Verification items for the finished model (mm, model axes). Face numbers are marked on the shaded views. A direction names the side the tool comes from. Round coordinates to 2 decimals unless told otherwise and drop trailing zeros. Loops run counter-clockwise (first coordinate to the right, second up) from the corner with the lowest first, then second, coordinate; pieces in that order, holes last. Notation, with made-up numbers: (68, -33.75) - (104, -33.75) arc R30 cw to (104, -10.75) - close; hole circle Ø4 at (43, 72). An arc over 180 degrees is marked (long way). Use a Markdown table: item, result. Add a question column.
```python
from build123d import *

# Parameters (mm, degrees)
F0_W          = 44.7
F0_H          = 40.1
F0_R          = 5
F1_DEPTH      = 8
F0_R_2        = 4
F2_DEPTH      = 1
F3_R          = 7.5
F4_DEPTH      = 25
F5_W          = 3.2212789527
F5_H          = 14.6500294167
F6_DEPTH      = 25
F7_R          = 5.5
F8_DEPTH      = 10
F9_R          = 5
F10_T4_DEPTH  = 14.6500294167
F10_S5_R      = 7.5
F10_T6_DEPTH  = 10
F10_T10_DEPTH = 14.6500294167
F10_S11_R     = 7.5
F10_T12_DEPTH = 10


# Not quite as in the source:
# - a fillet or chamfer that OpenCascade refuses, or shapes differently, is made with other operations: its cross-section is extruded or revolved along the edge and cut away or added


with BuildPart() as f1:
    # F0 (on Top) → F1 (new body)
    with BuildSketch(Plane.XY):
        Rectangle(F0_W, F0_H)
        with Locations((-15.35, -12.05)):
            Circle(F0_R, mode=Mode.SUBTRACT)
        with Locations((15.35, -12.05)):
            Circle(F0_R, mode=Mode.SUBTRACT)
        with Locations((-15.35, 12.05)):
            Circle(F0_R, mode=Mode.SUBTRACT)
        with Locations((15.35, 12.05)):
            Circle(F0_R, mode=Mode.SUBTRACT)
    extrude(amount=F1_DEPTH)

    # F0 (on Top) → F2 (join)
    with BuildSketch(Plane.XY):
        with Locations((15.35, 12.05)):
            Circle(F0_R)
        with Locations((15.35, 12.05)):
            Circle(F0_R_2, mode=Mode.SUBTRACT)
        with Locations((15.35, -12.05)):
            Circle(F0_R)
        with Locations((15.35, -12.05)):
            Circle(F0_R_2, mode=Mode.SUBTRACT)
        with Locations((-15.35, -12.05)):
            Circle(F0_R)
        with Locations((-15.35, -12.05)):
            Circle(F0_R_2, mode=Mode.SUBTRACT)
        with Locations((-15.35, 12.05)):
            Circle(F0_R)
        with Locations((-15.35, 12.05)):
            Circle(F0_R_2, mode=Mode.SUBTRACT)
    extrude(amount=F2_DEPTH)

    # F3 (on face) → F4 (join)
    with BuildSketch(Plane.XY.offset(8)):
        Circle(F3_R)
    extrude(amount=F4_DEPTH)

    # F5 (on face) → F6 (join)
    with BuildSketch(Plane.XY.offset(33)):
        Rectangle(F5_W, F5_H)
    extrude(amount=F6_DEPTH)

    # F7 (on face) → F8 (cut)
    with BuildSketch(Plane(origin=(-1.6106394764, 0, 0), x_dir=(0, -1, 0), z_dir=(-1, 0, 0))):
        with Locations((0, 45.5)):
            Circle(F7_R)
    extrude(amount=-F8_DEPTH, mode=Mode.SUBTRACT)

    # F9
    f9_edges = [f1.edges().sort_by_distance(p)[0] for p in [
        (0, 7.325015, 58),
        (0, -7.325015, 58),
        (-22.35, 20.05, 4),
        (-22.35, -20.05, 4),
        (22.35, -20.05, 4),
        (22.35, 20.05, 4),
    ]]
    fillet(f9_edges, radius=F9_R)

    # F10: fillet of radius 5 on 3 edges, made by hand


with BuildPart() as f10_tool2:
    # F10_s3 → F10_t4 (new body)
    with BuildSketch(Plane.XZ.offset(7.3250147083)):
        with BuildLine():
            ThreePointArc((6.6106394764, 33), (3.0751055704, 34.4644660941), (1.6106394764, 38))
            Line((1.6106394764, 38), (1.6106394764, 33))
            Line((1.6106394764, 33), (6.6106394764, 33))
        make_face()
    extrude(amount=-F10_T4_DEPTH)

    # F10_s5 → F10_t6 (intersect, symmetric)
    with BuildSketch(Plane.XY.offset(35.5)):
        Circle(F10_S5_R)
    extrude(amount=F10_T6_DEPTH, both=True, mode=Mode.INTERSECT)


with BuildPart() as f1_1:
    add(f1.part)

    # F10_t1: union F10_tool2
    add(f10_tool2.part)


with BuildPart() as f10_tool8:
    # F10_s9 → F10_t10 (new body)
    with BuildSketch(Plane.XZ.offset(-7.3250147083)):
        with BuildLine():
            ThreePointArc((-6.6106394764, 33), (-3.0751055704, 34.4644660941), (-1.6106394764, 38))
            Line((-1.6106394764, 38), (-1.6106394764, 33))
            Line((-1.6106394764, 33), (-6.6106394764, 33))
        make_face()
    extrude(amount=F10_T10_DEPTH)

    # F10_s11 → F10_t12 (intersect, symmetric)
    with BuildSketch(Plane.XY.offset(35.5)):
        Circle(F10_S11_R)
    extrude(amount=F10_T12_DEPTH, both=True, mode=Mode.INTERSECT)


with BuildPart() as f1_2:
    add(f1_1.part)

    # F10_t7: union F10_tool8
    add(f10_tool8.part)

    # F10_s13 → F10_t14 (revolve)
    with BuildSketch(Plane.XZ):
        with BuildLine():
            ThreePointArc((12.5, 8), (8.9644660941, 9.4644660941), (7.5, 13))
            Line((7.5, 13), (7.5, 8))
            Line((7.5, 8), (12.5, 8))
        make_face()
    revolve(axis=Axis((0, 0, 8), (0, 0, 1)))


solid = f1_2.part
```
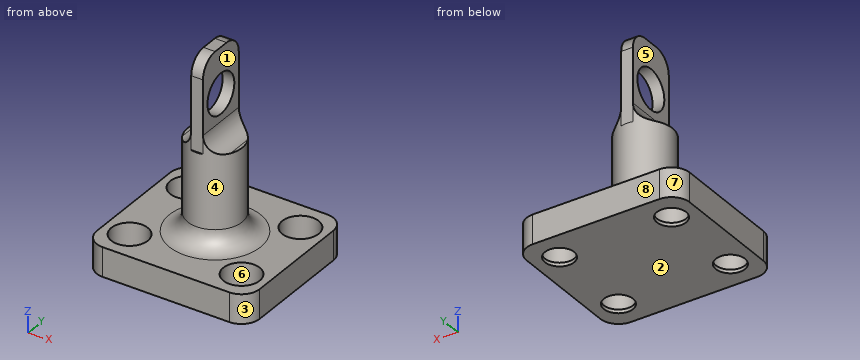
Q1. Release check for a two-part mould opening along X. For the marked faces 6, 7 and 8 record: +X half, -X half, draft (parallel to the pull), parting line (faces both ways), or undercut.
Q2. Go/stop test with flat-tipped pins: pin 1 Ø11.5 at (y, z) = (2, 51) entering from -X; pin 2 Ø1 at (y, z) = (-7, 41) entering from +X; pin 3 Ø1 at (x, y) = (-7, 1.5) entering from +Z. Record where each tip stops, or that it passes through.
Q3. Section check D-D on x = 0. Record the cut outline in (y, z).
Q4. Set-up check for the marked faces 1, 2, 3, 4 and 5: record each of +Z, -Z, +X, -X, +Y, -Y from which the full face is reachable in a straight line by a thin tool's end or side.
Q5. Thickness scan on line 1 along Y through (x, z) = (-15.35, 0.55); line 2 along Y through (x, z) = (-15.35, 6.75); line 3 along Z through (x, y) = (0.2, 0). Record the ranges inside material, lowest first.
Q6. Section check A-A on y = 0. Record the cut outline in (x, z).
Q7. Section check B-B on z = 45.5. Record the cut outline in (x, y).
Q8. Section check C-C on x = 15.35. Record the cut outline in (y, z), plus the area to 3 significant figures.
Determined:
| question | item | result |
|---|---|---|
| 1 | face 6 | undercut |
| 1 | face 7 | -X half |
| 1 | face 8 | draft |
| 2 | pin 1 | stops at x = -1.61 |
| 2 | pin 2 | stops at x = 1.61 |
| 2 | pin 3 | stops at z = 33 |
| 3 | outline | (-20.05, 0) - (20.05, 0) - (20.05, 8) - (12.5, 8) arc R5 cw to (7.5, 13) - (7.5, 33) - (7.33, 33) - (7.33, 53) arc R5 ccw to (2.33, 58) - (-2.33, 58) arc R5 ccw to (-7.33, 53) - (-7.33, 33) - (-7.5, 33) - (-7.5, 13) arc R5 cw to (-12.5, 8) - (-20.05, 8) - close; hole circle Ø11 at (0, 45.5) |
| 4 | face 1 | +Z, +X, +Y, -Y |
| 4 | face 2 | -Z, +X, -X, +Y, -Y |
| 4 | face 3 | +Z, -Z, +X, -Y |
| 4 | face 4 | +Z |
| 4 | face 5 | +Z, -X, +Y, -Y |
| 5 | line 1 | y = -20.05 to -16.05, -8.05 to 8.05, 16.05 to 20.05 |
| 5 | line 2 | y = -20.05 to -17.05, -7.05 to 7.05, 17.05 to 20.05 |
| 5 | line 3 | z = 0 to 40, 51 to 58 |
| 6 | outline | (-22.35, 0) - (22.35, 0) - (22.35, 8) - (12.5, 8) arc R5 cw to (7.5, 13) - (7.5, 33) - (6.61, 33) arc R5 cw to (1.61, 38) - (1.61, 40) - (-1.61, 40) - (-1.61, 38) arc R5 cw to (-6.61, 33) - (-7.5, 33) - (-7.5, 13) arc R5 cw to (-12.5, 8) - (-22.35, 8) - close; (-1.61, 51) - (1.61, 51) - (1.61, 58) - (-1.61, 58) - close |
| 7 | outline | (-1.61, -7.33) - (1.61, -7.33) - (1.61, -5.5) - (-1.61, -5.5) - close; (-1.61, 5.5) - (1.61, 5.5) - (1.61, 7.33) - (-1.61, 7.33) - close |
| 8 | outline | (-20.05, 0) - (-16.05, 0) - (-16.05, 1) - (-17.05, 1) - (-17.05, 8) - (-20.05, 8) - close; (-8.05, 0) - (8.05, 0) - (8.05, 1) - (7.05, 1) - (7.05, 8) - (-7.05, 8) - (-7.05, 1) - (-8.05, 1) - close; (16.05, 0) - (20.05, 0) - (20.05, 8) - (17.05, 8) - (17.05, 1) - (16.05, 1) - close |
| 8 | area | 165 mm² |
